Geometry check sheet. Reference: the model listing, model coordinates, mm. A direction names the side the tool comes from. Coordinates: 2 decimals unless noted, no trailing zeros. Order: outer loops, then holes, each group sorted by start corner. A loop starts at its lowest first (then second) coordinate and runs counter-clockwise, first axis right, second up. Notation, with made-up numbers: (71.25, -30) -> (107.25, -30) arc R31 cw to (107.25, -6) -> close; hole circle Ø11 at (48, 42.25). An arc over 180 degrees is marked (long way). Answer as CSV lines item,"result". Start each with the question number.
from build123d import *

# Parameters (mm, degrees)
SKETCH2_W           = 46
SKETCH2_H           = 46
BOSS_EXTRUDE1_DEPTH = 5
SKETCH4_R           = 4.1
CUT_EXTRUDE2_DEPTH  = 3
SKETCH5_R           = 2.1
CUT_EXTRUDE4_DEPTH  = 6
SKETCH6_R           = 1.6
CUT_EXTRUDE5_DEPTH  = 5


with BuildPart() as part:
    # Sketch2 → Boss-Extrude1 (new body)
    with BuildSketch(Plane(origin=(0, 0, 0), x_dir=(1, 0, 0), z_dir=(0, 1, 0))):
        Rectangle(SKETCH2_W, SKETCH2_H)
    extrude(amount=BOSS_EXTRUDE1_DEPTH)

    # Sketch4 → Cut-Extrude2 (cut)
    with BuildSketch(Plane(origin=(0, 0, 0), x_dir=(1, 0, 0), z_dir=(0, 1, 0))):
        Circle(SKETCH4_R)
    extrude(amount=CUT_EXTRUDE2_DEPTH, mode=Mode.SUBTRACT)

    # Sketch5 → Cut-Extrude4 (cut, through all)
    with BuildSketch(Plane(origin=(0, 0, 0), x_dir=(1, 0, 0), z_dir=(0, 1, 0))):
        Circle(SKETCH5_R)
    extrude(amount=CUT_EXTRUDE4_DEPTH, mode=Mode.SUBTRACT)

    # Sketch6 → Cut-Extrude5 (cut)
    with BuildSketch(Plane(origin=(0, 0, 0), x_dir=(1, 0, 0), z_dir=(0, 1, 0))):
        with Locations((18.12, 19.125)):
            Circle(SKETCH6_R)
        with Locations((-18.12, 19.125)):
            Circle(SKETCH6_R)
        with Locations((-18.12, -19.125)):
            Circle(SKETCH6_R)
        with Locations((18.12, -19.125)):
            Circle(SKETCH6_R)
    extrude(amount=CUT_EXTRUDE5_DEPTH, mode=Mode.SUBTRACT)


solid = part.part
Q1. Sectioned sample at C-C, the plane y = 0.75. Record the cut outline in (x, z) (3 decimals), then the cut area to 3 significant figures.
Q2. Release check for a two-part mould opening along Z. For faces 3 (the flat face through (2, 3, 2)), 4 (the flat face through (-23, 2, 0)), 5 (the flat face through (0, 2, -23)), 6 (the flat face through (0, 2, 23)) record: released by +Z, released by -Z, zero draft, split by the parting line, or undercut.
Q3. Sectioned sample at D-D, the plane y = 4.1. Record the cut outline in (x, z) (3 decimals), then the cut area to 3 significant figures.
Q4. Sectioned sample at A-A, the plane x = 18.12. Record the cut outline in (y, z) (3 decimals).
Q5. Go/stop test with flat-tipped pins: pin 1 Ø5 at (x, z) = (-13, 14.5) entering from -Y; pin 2 Ø1.9 at (x, z) = (18.12, -19.125) entering from +Y. Record where each tip stops, or that it passes through.
Q6. Thickness scan on L1, parallel to Z at x = -18.12, y = 1.7 (3 decimals); L2, parallel to X at y = 4.4, z = -19; L3, parallel to X at y = 4.6, z = -19.5. Record the ranges inside material, lowest first.
Q7. Sectioned sample at B-B, the plane x = 0. Record the cut outline in (y, z), then the cut area to 3 significant figures.
Q8. Access from +Z, -Z, +X, -X, +Y, -Y to the whole of each face (thin tool, end or side, straight path). Record for faces 1 (the cylindrical face through (18.98, 2.465, -20.474)), 2 (the cylindrical face through (-0.534, 1.479, -4.065)).
Geometry results:
1,outline,"(-23, -23) -> (23, -23) -> (23, 23) -> (-23, 23) -> close; hole circle Ø3.2 at (-18.12, -19.125); hole circle Ø3.2 at (-18.12, 19.125); hole circle Ø8.2 at (0, 0); hole circle Ø3.2 at (18.12, -19.125); hole circle Ø3.2 at (18.12, 19.125)"
1,area,"2,030 mm^2"
2,face 3,"undercut"
2,face 4,"zero draft"
2,face 5,"released by -Z"
2,face 6,"released by +Z"
3,outline,"(-23, -23) -> (23, -23) -> (23, 23) -> (-23, 23) -> close; hole circle Ø3.2 at (-18.12, -19.125); hole circle Ø3.2 at (-18.12, 19.125); hole circle Ø4.2 at (0, 0); hole circle Ø3.2 at (18.12, -19.125); hole circle Ø3.2 at (18.12, 19.125)"
3,area,"2,070 mm^2"
4,outline,"(0, -23) -> (5, -23) -> (5, -20.725) -> (0, -20.725) -> close; (0, -17.525) -> (5, -17.525) -> (5, 17.525) -> (0, 17.525) -> close; (0, 20.725) -> (5, 20.725) -> (5, 23) -> (0, 23) -> close"
5,pin 1,"stops at y = 0"
5,pin 2,"passes through"
6,L1,"z = -23 to -20.725, -17.525 to 17.525, 20.725 to 23"
6,L2,"x = -23 to -19.72, -16.52 to 16.52, 19.72 to 23"
6,L3,"x = -23 to -19.68, -16.56 to 16.56, 19.68 to 23"
7,outline,"(0, -23) -> (5, -23) -> (5, -2.1) -> (3, -2.1) -> (3, -4.1) -> (0, -4.1) -> close; (0, 4.1) -> (3, 4.1) -> (3, 2.1) -> (5, 2.1) -> (5, 23) -> (0, 23) -> close"
7,area,"197 mm^2"
8,face 1,"+Y, -Y"
8,face 2,"-Y"
